Autodesk Inventor part; units mm, degrees
ref_plane "YZ Plane" through (0, 0, 0) normal (1, 0, 0) x (0, 1, 0)
ref_plane "XZ Plane" through (0, 0, 0) normal (0, 1, 0) x (-1, 0, 0)
ref_plane "XY Plane" through (0, 0, 0) normal (0, 0, 1) x (1, 0, 0)
sketch "Sketch1" plane through (0, 0, 0) normal (0, 0, 1) x (1, 0, 0)
  line L0 (0, 9.3) -> (-0.425, 9.3)
  line L1 (-0.425, 9.3) -> (-0.425, 12.5)
  line L2 (-0.425, 12.5) -> (-0.635, 12.5)
  line L3 (-0.635, 12.5) -> (-0.635, 0)
  line L4 (-0.635, 0) -> (-0.425, 0)
  line L5 (-0.425, 0) -> (-0.425, 4)
  line L6 (-0.425, 4) -> (0, 4)
  line L7 (0, 4) -> (0, 9.3)
  point P0 (0, 0)
  dimension "d0" = 0.635
  dimension "d1" = 12.5
  dimension "d2" = 4
  dimension "d3" = 3.2
  dimension "d4" = 0.425
revolve "Revolution1" add sketch "Sketch1" angle 360 about axis through (0, 4, 0) along (0, 1, 0)
sketch "Sketch2" plane through (0, 0, 0) normal (1, 0, 0) x (0, 1, 0)
  line L0 (9.3, -0.425) -> (9.3, 0.425)
  line L1 (9.3, -0.1) -> (12.5, -0.1)
  line L2 (12.5, -0.425) -> (12.5, 0.425)
  line L3 (9.3, 0.1) -> (12.5, 0.1)
  line L4 (9.3, -0.1) -> (9.3, 0.1)
  line L5 (12.5, -0.1) -> (12.5, 0.1)
  point P0 (0, 0)
  dimension "d6" = 0.2
  dimension "d7" = 0.1
extrude "Extrusion1" cut sketch "Sketch2" along normal through all both and the other way through all
sketch "Sketch3" plane through (0, 0, 0) normal (1, 0, 0) x (0, 1, 0)
  line L0 (0, 0) -> (2, 0)
  line L1 (0, 0.635) -> (12.5, 0.635)
  line L2 (2, 0) -> (2, 0.635)
  line L3 (0, -0.635) -> (0, 0.635)
  line L4 (0, 0) -> (0, 0.635)
  line L5 (2, 0.635) -> (0, 0.635)
  dimension "d10" = 2
extrude "Extrusion2" cut sketch "Sketch3" along normal through all both and the other way through all
properties part number "SMA-PanelMount-Ni-AuPlated-Pin" material "Brass"
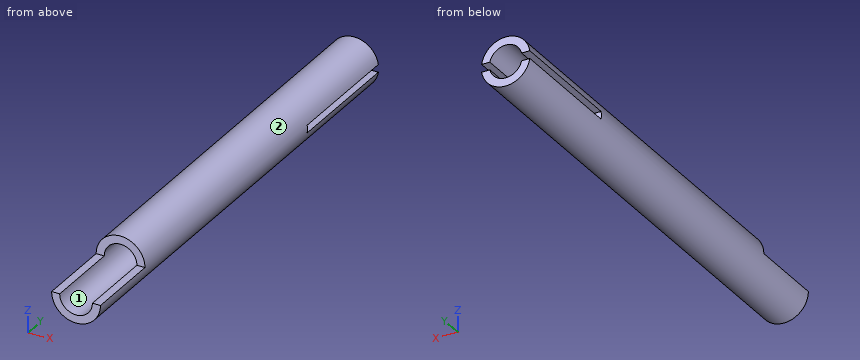
Geometry check sheet. Reference: the model listing, model coordinates, mm. Face numbers are marked on the shaded views. Round coordinates to 2 decimals unless told otherwise and drop trailing zeros. Order: outer loops, then holes, each group sorted by start corner. A loop starts at its lowest first (then second) coordinate and runs counter-clockwise, first axis right, second up. Notation, with made-up numbers: (-17, 45) - (12, 45) arc R24 cw to (12, 76) - close; hole circle Ø9 at (25, 74). An arc over 180 degrees is marked (long way). Use a Markdown table: item, result. Add a question column.
1) Section check D-D (y = 1). Record the cut outline in (x, z) (3 decimals).
2) Section check C-C (y = 5.5). Record the cut outline in (x, z) (3 decimals).
3) Mould release check, pull along X, two halves, no side actions. Record for the marked faces 1 and 2: released by +X, released by -X, zero draft, split by the parting line, or undercut.
4) Section check B-B (y = 2.75). Record the cut outline in (x, z) (3 decimals), then the cut area to 3 significant figures.
5) Section check A-A (x = 0). Record the cut outline in (y, z) (3 decimals).
6) Thickness scan on line 1 along X through (y, z) = (2.6, 0) (3 decimals); line 2 along Z through (x, y) = (0, 1.3) (3 decimals). Record the ranges inside material, lowest first.
7) Gauge pin test, flat ends, axial feed: P1, Ø0.7, axis at x = 0.5, z = 0, coming from the +Y side; P2, Ø0.7, axis at x = 0, z = 0.5, coming from the -Y side. Record the tip position at first contact, or that the pin passes through.
Established:
| question | item | result |
|---|---|---|
| 1 | outline | (-0.635, 0) arc R0.635 ccw to (0.635, 0) - (0.425, 0) arc R0.425 cw to (-0.425, 0) - close |
| 2 | outline | circle Ø1.27 at (0, 0) |
| 3 | face 1 | undercut |
| 3 | face 2 | split by the parting line |
| 4 | outline | circle Ø1.27 at (0, 0); hole circle Ø0.85 at (0, 0) |
| 4 | area | 0.699 mm2 |
| 5 | outline | (0, -0.635) - (12.5, -0.635) - (12.5, -0.425) - (9.3, -0.425) - (9.3, 0.425) - (12.5, 0.425) - (12.5, 0.635) - (2, 0.635) - (2, 0.425) - (4, 0.425) - (4, -0.425) - (0, -0.425) - close |
| 6 | line 1 | -0.635 to -0.425, 0.425 to 0.635 |
| 6 | line 2 | -0.635 to -0.425 |
| 7 | P1 | y = 12.5 |
| 7 | P2 | y = 2 |
